Answer from the drawing. Dimensions are ordinates in mm from the lowest x, y and z of the part. Coordinates: 2 decimals unless noted, no trailing zeros. Loops run counter-clockwise (first coordinate to the right, second up) from the corner with the lowest first, then second, coordinate; pieces in that order, holes last.
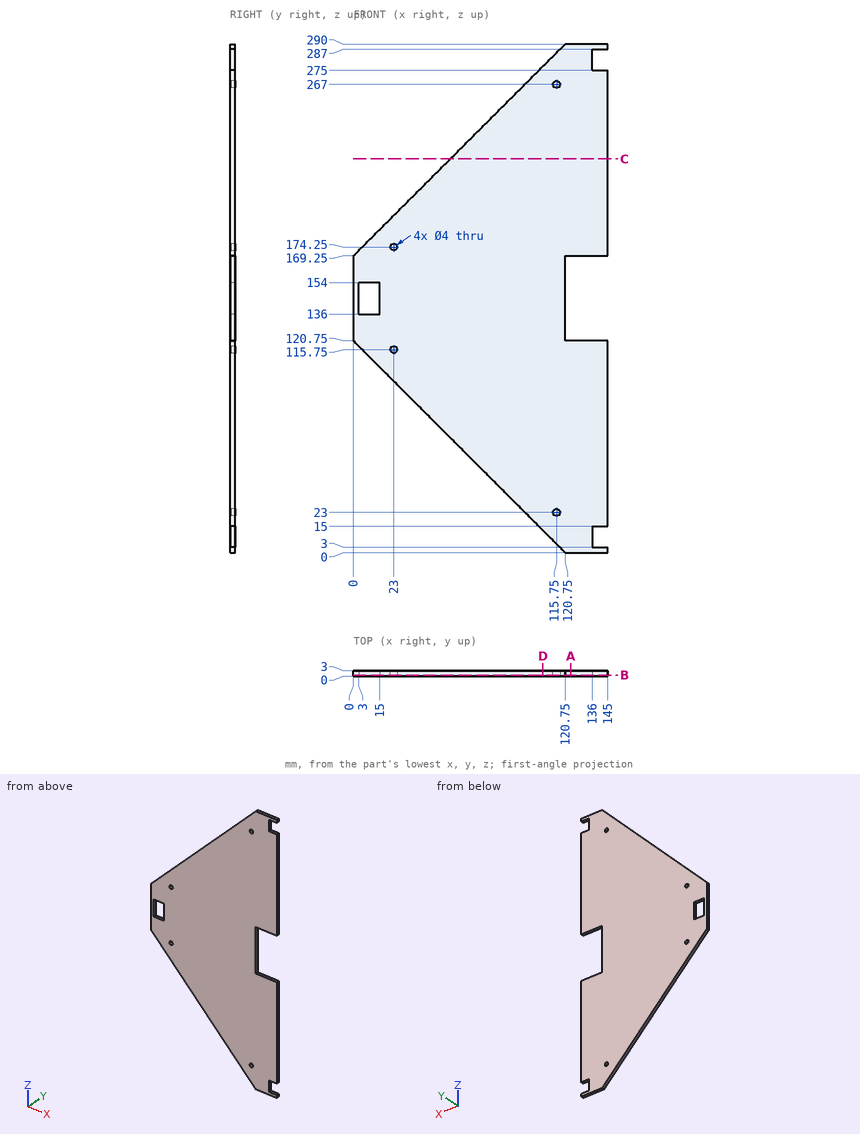
Item 1: A cutting plane is placed at B-B on y = 0.55. Determine the outline of the cut face in (x, z), then the cut area to 3 significant figures.
Numbers:
outline: (0, 120.75) - (120.75, 0) - (145, 0) - (145, 3) - (136, 3) - (136, 15) - (145, 15) - (145, 120.75) - (120.75, 120.75) - (120.75, 169.25) - (145, 169.25) - (145, 275) - (136, 275) - (136, 287) - (145, 287) - (145, 290) - (120.75, 290) - (0, 169.25) - close; hole (3, 136) - (15, 136) - (15, 154) - (3, 154) - close; hole circle Ø4 at (23, 115.75); hole circle Ø4 at (23, 174.25); hole circle Ø4 at (115.75, 23); hole circle Ø4 at (115.75, 267)
area: 25,800 mm2
Item 2: A cutting plane is placed at A-A on x = 124. Determine the outline of the cut face in (y, z), then the cut area to 4 significant figures.
Numbers:
outline: (0, 0) - (3, 0) - (3, 120.75) - (0, 120.75) - close; (0, 169.25) - (3, 169.25) - (3, 290) - (0, 290) - close
area: 724.5 mm2
Item 3: Find the intervals of material crossed by line 1 along X through (y, z) = (2.8, 152); line 2 along Z through (x, y) = (22, 0.4); line 3 along Z through (x, y) = (123, 2.15), in increasing order.
Numbers:
line 1: x = 0 to 3, 15 to 120.75
line 2: z = 98.75 to 114.02, 117.48 to 172.52, 175.98 to 191.25
line 3: z = 0 to 120.75, 169.25 to 290
Item 4: A cutting plane is placed at C-C on z = 224.5. Determine the outline of the cut face in (x, y).
Numbers:
outline: (55.25, 0) - (145, 0) - (145, 3) - (55.25, 3) - close
Item 5: A cutting plane is placed at D-D on x = 108. Determine the outline of the cut face in (y, z).
Numbers:
outline: (0, 12.75) - (3, 12.75) - (3, 277.25) - (0, 277.25) - close
Item 6: Given pin 1 (1.5 mm diameter, centred on x = 10.5, y = 2, fed in from -Z); pin 2 (1.5 mm diameter, centred on x = 11, y = 1.5, fed in from +Z); pin 3 (1.5 mm diameter, centred on y = 2, z = 137, fed in from +X), each flat-ended and moving along its own axis, determine where each tip first touches the part or whether it passes through.
Numbers:
pin 1: stops at z = 109.5
pin 2: stops at z = 181
pin 3: stops at x = 120.75
